from build123d import *

# Parameters (mm, degrees)
SKETCH1_R           = 15
SKETCH1_R_2         = 2
BOSS_EXTRUDE1_DEPTH = 3
SKETCH2_R           = 1.5
CUT_EXTRUDE1_DEPTH  = 3
CHAMFER1_SIZE       = 2
SKETCH3_R           = 1.3
CUT_EXTRUDE2_DEPTH  = 3


with BuildPart() as part:
    # Sketch1 → Boss-Extrude1 (new body)
    with BuildSketch(Plane(origin=(0, 0, 0), x_dir=(1, 0, 0), z_dir=(0, 1, 0))):
        with Locations(Location((0, 0, 0), (0, 0, 270))):
            Circle(SKETCH1_R)
        with Locations(Location((0, 0, 0), (0, 0, 270))):
            Circle(SKETCH1_R_2, mode=Mode.SUBTRACT)
    extrude(amount=BOSS_EXTRUDE1_DEPTH)

    # Sketch2 → Cut-Extrude1 (cut)
    with BuildSketch(Plane(origin=(0, 3, 0), x_dir=(1, 0, 0), z_dir=(0, 1, 0))):
        with Locations(Location((6, 0, 0), (0, 0, 270))):
            Circle(SKETCH2_R)
        with Locations(Location((-6, 0, 0), (0, 0, 270))):
            Circle(SKETCH2_R)
    extrude(amount=-CUT_EXTRUDE1_DEPTH, mode=Mode.SUBTRACT)

    # Chamfer1
    chamfer1_edges = [part.edges().sort_by_distance(p)[0] for p in [
        (6, 3, -1.5),
        (-6, 3, -1.5),
    ]]
    chamfer(chamfer1_edges, length=CHAMFER1_SIZE)

    # Sketch3 → Cut-Extrude2 (cut)
    with BuildSketch(Plane(origin=(0, 3, 0), x_dir=(1, 0, 0), z_dir=(0, 1, 0))):
        with Locations(Location((-7.072135785, 7.072135785, 0), (0, 0, 270))):
            Circle(SKETCH3_R)
        with Locations(Location((7.072135785, 7.072135785, 0), (0, 0, 270))):
            Circle(SKETCH3_R)
        with Locations(Location((7.072135785, -7.072135785, 0), (0, 0, 270))):
            Circle(SKETCH3_R)
        with Locations(Location((-7.072135785, -7.072135785, 0), (0, 0, 270))):
            Circle(SKETCH3_R)
    extrude(amount=-CUT_EXTRUDE2_DEPTH, mode=Mode.SUBTRACT)


solid = part.part
Verification items for the finished model (mm, model axes). Coordinates: 2 decimals unless noted, no trailing zeros. Write each loop counter-clockwise with the first axis right and the second up, starting at its lowest first coordinate (ties: lowest second). Pieces come first, ordered by that corner, then holes. Notation, with made-up numbers: (-2, -33) - (27, -33) arc R26 ccw to (27, -5) - close; hole circle Ø8 at (-23.5, 85.5). An arc over 180 degrees is marked (long way). Answer as a JSON object with one key per item and string values.
(1) Thickness scan on line 1 along X through (y, z) = (0.7, 0); line 2 along Z through (x, y) = (-6, 1.3); line 3 along X through (y, z) = (2.1, 0). Record the ranges inside material, lowest first.
Report:
{"line 1": "-15 to -7.5, -4.5 to -2, 2 to 4.5, 7.5 to 15", "line 2": "-13.75 to -7.81, -6.34 to -1.8, 1.8 to 6.34, 7.81 to 13.75", "line 3": "-15 to -8.6, -3.4 to -2, 2 to 3.4, 8.6 to 15"}
(2) Cross-section at A-A on x = 0. Record the cut outline in (y, z).
Report:
{"outline": "(0, -15) - (3, -15) - (3, -2) - (0, -2) - close; (0, 2) - (3, 2) - (3, 15) - (0, 15) - close"}
(3) Cross-section at B-B on z = 0. Record the cut outline in (x, y).
Report:
{"outline": "(-15, 0) - (-7.5, 0) - (-7.5, 1) - (-9.5, 3) - (-15, 3) - close; (-4.5, 0) - (-2, 0) - (-2, 3) - (-2.5, 3) - (-4.5, 1) - close; (2, 0) - (4.5, 0) - (4.5, 1) - (2.5, 3) - (2, 3) - close; (7.5, 0) - (15, 0) - (15, 3) - (9.5, 3) - (7.5, 1) - close"}
(4) Mould release check, pull along Z, two halves, no side actions. Record for faces 1 (the cylindrical face through (0.66, 1.479, -14.985)), 2 (the cylindrical face through (6.57, 1.52, 8.27)), 3 (the flat face through (0, 3, 3)): pulls with the +Z half, pulls with the -Z half, needs draft (parallel to the pull), parting line crosses it, or undercut.
Report:
{"face 1": "parting line crosses it", "face 2": "undercut", "face 3": "needs draft"}
(5) Cross-section at C-C on y = 2.65. Record the cut outline in (x, z), plus the area to 3 significant figures.
Report:
{"outline": "circle Ø30 at (0, 0); hole circle Ø6.3 at (-6, 0); hole circle Ø2.6 at (-7.07, -7.07); hole circle Ø2.6 at (-7.07, 7.07); hole circle Ø4 at (0, 0); hole circle Ø6.3 at (6, 0); hole circle Ø2.6 at (7.07, -7.07); hole circle Ø2.6 at (7.07, 7.07)", "area": "611 mm^2"}
(6) Cross-section at D-D on z = -9. Record the cut outline in (x, y), plus the area to 3 significant figures.
Report:
{"outline": "(-12, 0) - (12, 0) - (12, 3) - (-12, 3) - close", "area": "72.0 mm^2"}
(7) Gauge pin test, flat end, axial feed: pin 1 Ø1.5 at (y, z) = (2.5, 8) entering from +X. Record the tip position at first contact, or that the pin passes through.
Report:
{"pin 1": "x = 13.13"}
